from build123d import *

# Parameters (mm, degrees)
F0_R     = 4
F0_R_2   = 3
F0_R_3   = 10
F1_DEPTH = 4


with BuildPart() as f1:
    # F0 (on Top) → F1 (new body)
    with BuildSketch(Plane.XY):
        with BuildLine():
            ThreePointArc((0, 5), (1.464466, 1.464466), (5, 0))
            Line((5, 0), (55, 0))
            ThreePointArc((55, 0), (58.535534, 1.464466), (60, 5))
            Line((60, 5), (60, 29.188612))
            ThreePointArc((60, 29.188612), (59.929471, 30.025459), (59.719874, 30.838698))
            Line((59.719874, 30.838698), (29.719874, 116.650087))
            ThreePointArc((29.719874, 116.650087), (27.893922, 119.077403), (25, 120))
            Line((25, 120), (5, 120))
            ThreePointArc((5, 120), (1.464466, 118.535534), (0, 115))
            Line((0, 115), (0, 5))
        make_face()
        with Locations((15, 15)):
            Circle(F0_R, mode=Mode.SUBTRACT)
        with Locations((25, 15)):
            Circle(F0_R_2, mode=Mode.SUBTRACT)
        with Locations((15, 50)):
            Circle(F0_R_2, mode=Mode.SUBTRACT)
        with Locations((40, 15)):
            Circle(F0_R_2, mode=Mode.SUBTRACT)
        with Locations((50, 15)):
            Circle(F0_R, mode=Mode.SUBTRACT)
        with Locations((35.990281, 36.892906)):
            Circle(F0_R_3, mode=Mode.SUBTRACT)
        with Locations((35.990281, 56.421787)):
            Circle(F0_R, mode=Mode.SUBTRACT)
        with Locations((15, 60)):
            Circle(F0_R, mode=Mode.SUBTRACT)
        with Locations((15, 70)):
            Circle(F0_R_2, mode=Mode.SUBTRACT)
        with Locations((15, 97)):
            Circle(F0_R_2, mode=Mode.SUBTRACT)
        with Locations((15, 108)):
            Circle(F0_R, mode=Mode.SUBTRACT)
        with Locations((35.990281, 69.710411)):
            Circle(F0_R_2, mode=Mode.SUBTRACT)
    extrude(amount=F1_DEPTH)


solid = f1.part
Can you work these out from the model? Positions are in its coordinate system, mm. Coordinates: 2 decimals unless noted, no trailing zeros. Order: outer loops, then holes, each group sorted by start corner. A loop starts at its lowest first (then second) coordinate and runs counter-clockwise, first axis right, second up. Notation, with made-up numbers: (54.5, 58.5) -> (81.5, 58.5) arc R24 cw to (81.5, 75.5) -> close; hole circle Ø2 at (56, 42.25). An arc over 180 degrees is marked (long way). Use one line per item in the form item = value.
Q1. Imagine slicing it at D-D, the plane z = 3.4. Give the number of separate pieces and of enclosed holes in the cut face, then the cut area to 3 significant figures.
From the geometry:
separate_pieces = 1
enclosed_holes = 12
area = 5,030 mm²
Q2. Imagine slicing it at C-C, the plane x = 52.5. List the corners of the cut face in (y, z) for me, then the cut area to 3 significant figures.
From the geometry:
outline = (0, 0) -> (11.88, 0) -> (11.88, 4) -> (0, 4) -> close; (18.12, 0) -> (51.49, 0) -> (51.49, 4) -> (18.12, 4) -> close
area = 181 mm²
Q3. Will this pin go through, and if not, where does the flat tip stop? P1, Ø3.5, axis at x = 40, y = 15, coming from the -Z side.
From the geometry:
P1 = through
Q4. We'd pull the mould along Y, two halves only. Please class faces 1 (the face through (28, 119, 2)), 2 (the face through (14.133, 56.095, 1.972)), 3 (the face through (30, 0, 2)): released by +Y, released by -Y, zero draft, split by the parting line, or undercut.
From the geometry:
face_1 = released by +Y
face_2 = undercut
face_3 = released by -Y
Q5. Imagine slicing it at A-A, the plane y = 15. List the corners of the cut face in (x, z) for me, then the cut area to 3 significant figures.
From the geometry:
outline = (0, 0) -> (11, 0) -> (11, 4) -> (0, 4) -> close; (19, 0) -> (22, 0) -> (22, 4) -> (19, 4) -> close; (28, 0) -> (37, 0) -> (37, 4) -> (28, 4) -> close; (43, 0) -> (46, 0) -> (46, 4) -> (43, 4) -> close; (54, 0) -> (60, 0) -> (60, 4) -> (54, 4) -> close
area = 128 mm²
Q6. I need wall thicknesses on L1, parallel to X at y = 13.5, z = 1.95; L2, parallel to X at y = 98, z = 3.15; L3, parallel to X at y = 34, z = 0.7. Which ranges of each line are inside material? Lowest first, please.
From the geometry:
L1 = 0 to 11.29, 18.71 to 22.4, 27.6 to 37.4, 42.6 to 46.29, 53.71 to 60
L2 = 0 to 12.17, 17.83 to 36.24
L3 = 0 to 26.42, 45.56 to 58.61
Q7. Imagine slicing it at B-B, the plane x = 15. List the corners of the cut face in (y, z) for me, then the cut area to 3 significant figures.
From the geometry:
outline = (0, 0) -> (11, 0) -> (11, 4) -> (0, 4) -> close; (19, 0) -> (47, 0) -> (47, 4) -> (19, 4) -> close; (53, 0) -> (56, 0) -> (56, 4) -> (53, 4) -> close; (64, 0) -> (67, 0) -> (67, 4) -> (64, 4) -> close; (73, 0) -> (94, 0) -> (94, 4) -> (73, 4) -> close; (100, 0) -> (104, 0) -> (104, 4) -> (100, 4) -> close; (112, 0) -> (120, 0) -> (120, 4) -> (112, 4) -> close
area = 312 mm²
